Here's how the part is built. I have some questions about the finished solid (model axes, mm). A direction names the side the tool comes from. Coordinates: 2 decimals unless noted, no trailing zeros. Order: outer loops, then holes, each group sorted by start corner. A loop starts at its lowest first (then second) coordinate and runs counter-clockwise, first axis right, second up. Notation, with made-up numbers: (34.25, 6.5) - (40.25, 6.5) arc R26 cw to (40.25, 41.5) - close; hole circle Ø11 at (74.5, 51). An arc over 180 degrees is marked (long way). Answer in a Markdown table with one row per item. Add a question column.
Item 1: I want a section at B-B (x = -8.5). Please give me the cut outline in (y, z), plus the area to 3 significant figures.
Item 2: Thinking about a two-plate mould opening in Y: for faces 1 (the flat face through (-3.15, 1, 0)), 2 (the flat face through (0, -3, 0)), 3 (the cylindrical face through (-0.065, -1.504, -2.378)), which applies, +Y half, -Y half, draft (parallel to the pull), parting line (faces both ways), or undercut?
Item 3: Will these pins go through, and if not, where does the flat tip stop? pin 1 Ø3 at (x, z) = (6, -1.5) entering from +Y; pin 2 Ø0.8 at (x, y) = (0, 5.5) entering from -Z; pin 3 Ø2.5 at (x, z) = (-8.5, 0) entering from -Y; pin 4 Ø3 at (x, z) = (7.5, 0.5) entering from +Y.
Item 4: On a 3-axis mill with a long thin cutter (end or side, diameter ignored), from which of +Z, -Z, +X, -X, +Y, -Y can I reach the whole of each face in a straight line? I mean faces 4 (the cylindrical face through (-3.58, 5.51, -2.4)), 5 (the cylindrical face through (3.58, 5.51, -2.4)), 6 (the flat face through (-7.1, 1.6, 1.4)), 7 (the flat face through (0, 5.5, -3)). Say none if no direction works.
Item 5: I want a section at D-D (x = 0). Count the separate pieces of the cut face and the enclosed holes in it, plus the area to 4 significant figures.
Item 6: If I drill on line 1 along Y through (x, z) = (0, 3.3); line 2 along Y through (x, z) = (0, -2.5); line 3 along Z through (x, y) = (-2.5, 0), over which ranges is the centre line in solid material (lowest first)? Write a range as from..to.
Item 7: I want a section at A-A (y = 3). Please give me the cut outline in (x, z).
Item 8: I want a section at C-C (y = -3.5). Please give me the cut outline in (x, z).
```python
from build123d import *

# Parameters (mm, degrees)
SKIZZE1_W                                            = 25
SKIZZE1_H                                            = 10
AUFSATZ_LINEAR_AUSTRAGEN1_DEPTH                      = 4
STIRNSENKUNG_F_R_M3_ZYLINDERSCHRAUBE_MIT_D           = 3.4
STIRNSENKUNG_F_R_M3_ZYLINDERSCHRAUBE_MIT_CBORE_D     = 6.5
STIRNSENKUNG_F_R_M3_ZYLINDERSCHRAUBE_MIT_CBORE_DEPTH = 3.4
VERRUNDUNG1_R                                        = 3
SKIZZE4_W                                            = 6.3
SKIZZE4_H                                            = 1.6
SCHNITT_LINEAR_AUSTRAGEN1_DEPTH                      = 8
SKIZZE5_W                                            = 8.3
SKIZZE5_H                                            = 6
SKIZZE5_W_2                                          = 6.3
SKIZZE5_H_2                                          = 1.6
AUFSATZ_LINEAR_AUSTRAGEN2_DEPTH                      = 1
VERRUNDUNG2_R                                        = 2
SKIZZE6_R                                            = 0.5
SCHNITT_LINEAR_AUSTRAGEN2_DEPTH                      = 9
FASE1_SIZE                                           = 0.5


with BuildPart() as part:
    # Skizze1 → Aufsatz-Linear austragen1 (new body, symmetric)
    with BuildSketch(Plane.XY):
        Rectangle(SKIZZE1_W, SKIZZE1_H)
    extrude(amount=AUFSATZ_LINEAR_AUSTRAGEN1_DEPTH, both=True)

    # Stirnsenkung für M3 Zylinderschraube mit Innensechskant1 (through all)
    with Locations(Plane(origin=(0, 5, 0), x_dir=(1, 0, 0), z_dir=(0, 1, 0))):
        with Locations((-8.5, 0), (8.5, 0)):
            CounterBoreHole(STIRNSENKUNG_F_R_M3_ZYLINDERSCHRAUBE_MIT_D / 2, STIRNSENKUNG_F_R_M3_ZYLINDERSCHRAUBE_MIT_CBORE_D / 2, STIRNSENKUNG_F_R_M3_ZYLINDERSCHRAUBE_MIT_CBORE_DEPTH)

    # Verrundung1
    verrundung1_edges = [part.edges().sort_by_distance(p)[0] for p in [
        (12.5, 0, 4),
        (-12.5, 0, 4),
        (12.5, 0, -4),
        (-12.5, 0, -4),
    ]]
    fillet(verrundung1_edges, radius=VERRUNDUNG1_R)

    # Skizze4 → Schnitt-Linear austragen1 (cut)
    with BuildSketch(Plane(origin=(0, 5, 0), x_dir=(1, 0, 0), z_dir=(0, 1, 0))):
        Rectangle(SKIZZE4_W, SKIZZE4_H)
    extrude(amount=-SCHNITT_LINEAR_AUSTRAGEN1_DEPTH, mode=Mode.SUBTRACT)

    # Skizze5 → Aufsatz-Linear austragen2 (add)
    with BuildSketch(Plane(origin=(0, 5, 0), x_dir=(1, 0, 0), z_dir=(0, 1, 0))):
        Rectangle(SKIZZE5_W, SKIZZE5_H)
        Rectangle(SKIZZE5_W_2, SKIZZE5_H_2, mode=Mode.SUBTRACT)
    extrude(amount=AUFSATZ_LINEAR_AUSTRAGEN2_DEPTH)

    # Verrundung2
    verrundung2_edges = [part.edges().sort_by_distance(p)[0] for p in [
        (-4.15, 5.5, -3),
        (-4.15, 5.5, 3),
        (4.15, 5.5, 3),
        (4.15, 5.5, -3),
    ]]
    fillet(verrundung2_edges, radius=VERRUNDUNG2_R)

    # Skizze6 → Schnitt-Linear austragen2 (cut, through all)
    with BuildSketch(Plane.XY.offset(4)):
        with Locations((0, 3)):
            Circle(SKIZZE6_R)
        with Locations((0, -2)):
            Circle(SKIZZE6_R)
    extrude(amount=-SCHNITT_LINEAR_AUSTRAGEN2_DEPTH, mode=Mode.SUBTRACT)

    # Fase1
    fase1_edges = [part.edges().sort_by_distance(p)[0] for p in [
        (12.5, -5, 0),
        (0, -5, -4),
        (0, -5, 4),
        (-12.5, -5, 0),
        (-11.621320344, -5, 3.121320344),
        (-11.621320344, -5, -3.121320344),
        (11.621320344, -5, 3.121320344),
        (11.621320344, -5, -3.121320344),
    ]]
    chamfer(fase1_edges, length=FASE1_SIZE)


solid = part.part
```
Values follow:
| question | item | result |
|---|---|---|
| 1 | outline | (-5, -3.5) - (-4.5, -4) - (5, -4) - (5, -3.25) - (1.6, -3.25) - (1.6, -1.7) - (-5, -1.7) - close; (-5, 1.7) - (1.6, 1.7) - (1.6, 3.25) - (5, 3.25) - (5, 4) - (-4.5, 4) - (-5, 3.5) - close |
| 1 | area | 35.2 mm^2 |
| 2 | face 1 | draft |
| 2 | face 2 | +Y half |
| 2 | face 3 | undercut |
| 3 | pin 1 | stops at y = 5 |
| 3 | pin 2 | stops at z = -3 |
| 3 | pin 3 | passes through |
| 3 | pin 4 | stops at y = 1.6 |
| 4 | face 4 | -Z, -X, +Y |
| 4 | face 5 | -Z, +X, +Y |
| 4 | face 6 | +Y |
| 4 | face 7 | -Z, +X, -X, +Y |
| 5 | separate pieces | 5 |
| 5 | enclosed holes | 0 |
| 5 | area | 58.55 mm^2 |
| 6 | line 1 | y = -5..-2.5, -1.5..2.5, 3.5..5 |
| 6 | line 2 | y = -5..-2.5, -1.5..2.5, 3.5..6 |
| 6 | line 3 | z = -4..-0.8, 0.8..4 |
| 7 | outline | (-12.5, -1) arc R3 ccw to (-9.5, -4) - (-0.5, -4) - (-0.5, -0.8) - (-3.15, -0.8) - (-3.15, 0.8) - (-0.5, 0.8) - (-0.5, 4) - (-9.5, 4) arc R3 ccw to (-12.5, 1) - close; (0.5, -4) - (9.5, -4) arc R3 ccw to (12.5, -1) - (12.5, 1) arc R3 ccw to (9.5, 4) - (0.5, 4) - (0.5, 0.8) - (3.15, 0.8) - (3.15, -0.8) - (0.5, -0.8) - close; hole circle Ø6.5 at (-8.5, 0); hole circle Ø6.5 at (8.5, 0) |
| 8 | outline | (-12.5, -1) arc R3 ccw to (-9.5, -4) - (9.5, -4) arc R3 ccw to (12.5, -1) - (12.5, 1) arc R3 ccw to (9.5, 4) - (-9.5, 4) arc R3 ccw to (-12.5, 1) - close; hole circle Ø3.4 at (-8.5, 0); hole circle Ø3.4 at (8.5, 0) |
